```python
from build123d import *

# Parameters (mm, degrees)
SKETCH_1_W          = 47
SKETCH_1_H          = 106.16
SKETCH_1_W_2        = 10.5
SKETCH_1_H_2        = 10
EXTRUDE_1_DEPTH     = 3
SKETCH_4_R          = 1.5
SKETCH_4_W          = 47
SKETCH_4_H          = 5
CUT_EXTRUDE_2_DEPTH = 4
SKETCH_10_R         = 1.25
CUT_EXTRUDE_4_DEPTH = 10
SKETCH_16_W         = 17.5
SKETCH_16_H         = 2.5
CUT_EXTRUDE_5_DEPTH = 10
FILLET_1_R          = 3
CUT_EXTRUDE_7_DEPTH = 10
FILLET_2_R          = 1
FILLET_3_R          = 8
FILLET_4_R          = 3
FILLET_5_R          = 5
SKETCH_17_W         = 21
SKETCH_17_H         = 20
SKETCH_17_H_2       = 8
CUT_EXTRUDE_8_DEPTH = 10
FILLET_6_R          = 5
FILLET_7_R          = 2


# Some blends are built 0.0001 mm under size
with BuildPart() as part:
    # 草图1 → 凸台-拉伸1 (new body)
    with BuildSketch(Plane(origin=(0, 0, 0), x_dir=(1, 0, 0), z_dir=(0, 1, 0))):
        with Locations((0, -33.08)):
            Rectangle(SKETCH_1_W, SKETCH_1_H)
        with Locations((5.25, -13)):
            Rectangle(SKETCH_1_W_2, SKETCH_1_H_2, mode=Mode.SUBTRACT)
    extrude(amount=EXTRUDE_1_DEPTH)

    # 草图4 → 切除-拉伸2 (cut)
    with BuildSketch(Plane(origin=(0, 3, 0), x_dir=(1, 0, 0), z_dir=(0, 1, 0))):
        with Locations(Location((-14, -76.16, 0), (0, 0, 270))):
            Circle(SKETCH_4_R)
        with Locations(Location((14, -76.16, 0), (0, 0, 270))):
            Circle(SKETCH_4_R)
        with Locations((0, -83.66)):
            Rectangle(SKETCH_4_W, SKETCH_4_H)
    extrude(amount=-CUT_EXTRUDE_2_DEPTH, mode=Mode.SUBTRACT)

    # 草图10 → 切除-拉伸4 (cut)
    with BuildSketch(Plane(origin=(0, 3, 0), x_dir=(1, 0, 0), z_dir=(0, 1, 0))):
        with Locations(Location((13.5, 13.5, 0), (0, 0, 270))):
            Circle(SKETCH_10_R)
        with Locations(Location((13.5, -13.5, 0), (0, 0, 270))):
            Circle(SKETCH_10_R)
        with Locations(Location((-13.5, -13.5, 0), (0, 0, 270))):
            Circle(SKETCH_10_R)
        with Locations(Location((-13.5, 13.5, 0), (0, 0, 270))):
            Circle(SKETCH_10_R)
    extrude(amount=-CUT_EXTRUDE_4_DEPTH, mode=Mode.SUBTRACT)

    # 草图16 → 切除-拉伸5 (cut)
    with BuildSketch(Plane(origin=(0, 3, 0), x_dir=(1, 0, 0), z_dir=(0, 1, 0))):
        Polygon((-17.5, 17.5), (-17.5, 20), (-23.5, 20), (-23.5, -10), (-17.5, -10), align=None)
        Polygon((23.5, 20), (17.5, 20), (17.5, 17.5), (17.5, -10), (23.5, -10), align=None)
        with Locations((8.75, 18.75)):
            Rectangle(SKETCH_16_W, SKETCH_16_H)
        with Locations((-8.75, 18.75)):
            Rectangle(SKETCH_16_W, SKETCH_16_H)
    extrude(amount=-CUT_EXTRUDE_5_DEPTH, mode=Mode.SUBTRACT)

    # 圆角1
    fillet_1_edges = [part.edges().sort_by_distance(p)[0] for p in [
        (-17.5, 1.5, -17.5),
        (17.5, 1.5, -17.5),
        (23.5, 1.5, 10),
        (-23.5, 1.5, 10),
        (17.5, 1.5, 10),
        (-17.5, 1.5, 10),
    ]]
    fillet(fillet_1_edges, radius=FILLET_1_R - 0.0001)  # a hair under: the kernel refuses the full size

    # 草图9 → 切除-拉伸7 (cut)
    with BuildSketch(Plane(origin=(0, 3, 0), x_dir=(1, 0, 0), z_dir=(0, 1, 0))):
        Polygon((-3, -47.16), (-17.4375, -22.66), (-19, -22.66), (-19, -71.66), (-17.4375, -71.66), align=None)
        Polygon((0, -45.16), (13.258928571, -22.66), (-13.258928571, -22.66), align=None)
        Polygon((19, -22.66), (17.4375, -22.66), (3, -47.16), (17.4375, -71.66), (19, -71.66), align=None)
        Polygon((-13.258928571, -71.66), (13.258928571, -71.66), (0, -49.16), align=None)
    extrude(amount=-CUT_EXTRUDE_7_DEPTH, mode=Mode.SUBTRACT)

    # 圆角2
    # the kernel refuses this fillet: 1 mm, written as the material it adds along each edge
    with BuildSketch(Plane(origin=(-17.4375, 3, 71.66), x_dir=(-1, 0, 0), z_dir=(0, -1, 0)), Plane(origin=(17.4375, 3, 71.66), x_dir=(-0.507692307692314, 0, -0.8615384615384579), z_dir=(0, -1, 0)), Plane(origin=(17.4375, 3, 22.66), x_dir=(1, 0, 0), z_dir=(0, -1, 0)), Plane(origin=(-17.4375, 3, 22.66), x_dir=(0.5076923076923058, 0, 0.8615384615384627), z_dir=(0, -1, 0))) as fillet_2_piece_1:
        with BuildLine():
            CenterArc((FILLET_2_R * 0.571428571429, FILLET_2_R), FILLET_2_R, 210.510237406, 59.489762594)
            Line((-FILLET_2_R * 0.29010989011, FILLET_2_R * 0.492307692308), (0, 0))
            Line((0, 0), (FILLET_2_R * 0.571428571429, 0))
        make_face()
    extrude(amount=3)
    with BuildSketch(Plane(origin=(-19, 3, 71.66), x_dir=(0, 0, -1), z_dir=(0, -1, 0)), Plane(origin=(19, 3, 71.66), x_dir=(-1, 0, 0), z_dir=(0, -1, 0)), Plane(origin=(-19, 3, 22.66), x_dir=(1, 0, 0), z_dir=(0, -1, 0))) as fillet_2_piece_2:
        with BuildLine():
            CenterArc((FILLET_2_R, FILLET_2_R), FILLET_2_R, 180, 90)
            Line((0, FILLET_2_R), (0, 0))
            Line((0, 0), (FILLET_2_R, 0))
        make_face()
    extrude(amount=3)
    with BuildSketch(Plane(origin=(19, 3, 22.66), x_dir=(-1, 0, 0), z_dir=(0, -1, 0))) as fillet_2_piece_3:
        with BuildLine():
            CenterArc((FILLET_2_R, -FILLET_2_R), FILLET_2_R, 90, 90)
            Line((0, -FILLET_2_R), (0, 0))
            Line((0, 0), (FILLET_2_R, 0))
        make_face()
    extrude(amount=3)

    # 圆角3
    fillet_3_edges = [part.edges().sort_by_distance(p)[0] for p in [
        (3, 1.5, 47.16),
        (-3, 1.5, 47.16),
    ]]
    fillet(fillet_3_edges, radius=FILLET_3_R)

    # 圆角4
    fillet_4_edges = [part.edges().sort_by_distance(p)[0] for p in [
        (-13.258928571, 1.5, 22.66),
        (13.258928571, 1.5, 22.66),
        (0, 1.5, 45.16),
        (-13.258928571, 1.5, 71.66),
        (0, 1.5, 49.16),
        (13.258928571, 1.5, 71.66),
    ]]
    fillet(fillet_4_edges, radius=FILLET_4_R)

    # 圆角5
    fillet_5_edges = [part.edges().sort_by_distance(p)[0] for p in [
        (-23.5, 1.5, 81.16),
        (23.5, 1.5, 81.16),
    ]]
    fillet(fillet_5_edges, radius=FILLET_5_R)

    # 草图17 → 切除-拉伸8 (cut)
    with BuildSketch(Plane(origin=(0, 3, 0), x_dir=(1, 0, 0), z_dir=(0, 1, 0))):
        Rectangle(SKETCH_17_W, SKETCH_17_H)
        with Locations((0, -14)):
            Rectangle(SKETCH_17_W, SKETCH_17_H_2)
    extrude(amount=-CUT_EXTRUDE_8_DEPTH, mode=Mode.SUBTRACT)

    # 圆角6
    fillet_6_edges = [part.edges().sort_by_distance(p)[0] for p in [
        (-10.5, 1.5, 18),
        (-10.5, 1.5, -10),
        (10.5, 1.5, -10),
    ]]
    fillet(fillet_6_edges, radius=FILLET_6_R)

    # 圆角7
    fillet_7_edges = [part.edges().sort_by_distance(p)[0] for p in [
        (10.5, 1.5, 18),
    ]]
    fillet(fillet_7_edges, radius=FILLET_7_R)


solid = part.part
```
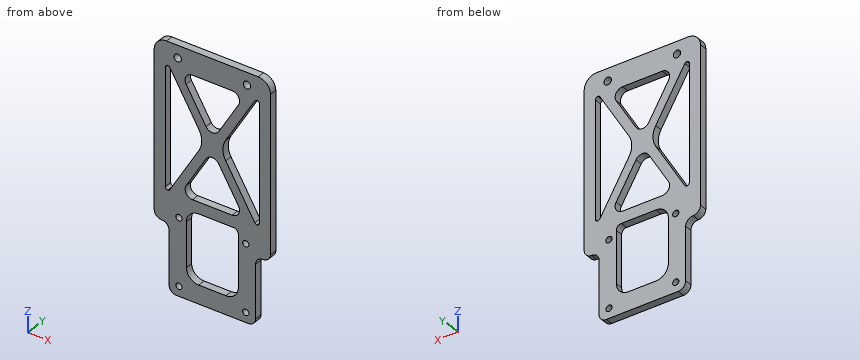
Verification items for the finished model (mm, model axes). Coordinates: 2 decimals unless noted, no trailing zeros. Loops run counter-clockwise (first coordinate to the right, second up) from the corner with the lowest first, then second, coordinate; pieces in that order, holes last. Notation, with made-up numbers: (-24.75, -26) - (30.25, -26) arc R26 cw to (30.25, 1) - close; hole circle Ø3 at (39, 17). An arc over 180 degrees is marked (long way). Answer as a JSON object with one key per item and string values.
(1) Cross-section at D-D, the plane z = 11. Record the boundary of the cut face in (x, y).
Response:
{"outline": "(-22.74, 0) - (-10.5, 0) - (-10.5, 3) - (-22.74, 3) - close; (10.5, 0) - (22.74, 0) - (22.74, 3) - (10.5, 3) - close"}
(2) Cross-section at A-A, the plane z = -13.5. Record the boundary of the cut face in (x, y), then the cut area to 3 significant figures.
Response:
{"outline": "(-17.5, 0) - (-14.75, 0) - (-14.75, 3) - (-17.5, 3) - close; (-12.25, 0) - (12.25, 0) - (12.25, 3) - (-12.25, 3) - close; (14.75, 0) - (17.5, 0) - (17.5, 3) - (14.75, 3) - close", "area": "90.0 mm²"}
(3) Scan lines: line 1 along X through (y, z) = (1.15, 76.16); line 2 along X through (y, z) = (0.8, -13.5); line 3 along X through (y, z) = (1.1, 33). Record each from-to range of solid material in increasing order.
Response:
{"line 1": "x = -23.5 to -15.5, -12.5 to 12.5, 15.5 to 23.5", "line 2": "x = -17.5 to -14.75, -12.25 to 12.25, 14.75 to 17.5", "line 3": "x = -23.5 to -19, -11.34 to -7.17, 7.17 to 11.34, 19 to 23.5"}
(4) Cross-section at B-B, the plane z = 32. Record the boundary of the cut face in (x, y) (3 decimals), then the cut area to 3 significant figures.
Response:
{"outline": "(-23.5, 0) - (-19, 0) - (-19, 3) - (-23.5, 3) - close; (-11.934, 0) - (-7.755, 0) - (-7.755, 3) - (-11.934, 3) - close; (7.755, 0) - (11.934, 0) - (11.934, 3) - (7.755, 3) - close; (19, 0) - (23.5, 0) - (23.5, 3) - (19, 3) - close", "area": "52.1 mm²"}
(5) Cross-section at C-C, the plane x = 1. Record the boundary of the cut face in (y, z).
Response:
{"outline": "(0, -17.5) - (3, -17.5) - (3, -10) - (0, -10) - close; (0, 18) - (3, 18) - (3, 22.66) - (0, 22.66) - close; (0, 42.08) - (3, 42.08) - (3, 52.24) - (0, 52.24) - close; (0, 71.66) - (3, 71.66) - (3, 81.16) - (0, 81.16) - close"}
(6) Go/stop test with flat-tipped pins: pin 1 Ø1.5 at (x, z) = (-13.5, 13.5) entering from -Y; pin 2 Ø1.5 at (y, z) = (1, 0) entering from +X. Record where each tip stops, or that it passes through.
Response:
{"pin 1": "passes through", "pin 2": "stops at x = 17.5"}
